Could you check a few things on this model? Use its own coordinates, in mm. A direction names the side the tool comes from. Coordinates: 2 decimals unless noted, no trailing zeros. Write each loop counter-clockwise with the first axis right and the second up, starting at its lowest first coordinate (ties: lowest second). Pieces come first, ordered by that corner, then holes. Notation, with made-up numbers: (82, 39.25) - (93, 39.25) arc R26 ccw to (93, 60.25) - close; hole circle Ø7 at (68.5, -25). An arc over 180 degrees is marked (long way). Write item = value, one per line. Start each with the question number.
```python
from build123d import *

# Parameters (mm, degrees)
BOSS_EXTRUDE1_DEPTH = 2.9972
SKETCH2_R           = 3
BOSS_EXTRUDE2_DEPTH = 11.176
SKETCH3_R           = 4.4958
BOSS_EXTRUDE3_DEPTH = 1.016
CUT_EXTRUDE1_DEPTH  = 1.524
SKETCH5_R           = 3.556
CUT_EXTRUDE2_DEPTH  = 1.9812
SKETCH6_R           = 1.1176
CUT_EXTRUDE3_DEPTH  = 32.262860272
SKETCH9_R           = 0.9906
CUT_EXTRUDE4_DEPTH  = 10.16


with BuildPart() as part:
    # Sketch1 → Boss-Extrude1 (new body)
    with BuildSketch(Plane(origin=(0, 0, 0), x_dir=(0, 0, -1), z_dir=(1, 0, 0))):
        with BuildLine():
            Line((24.769539012, 3.626266444), (5.771274976, 5.288399174))
            ThreePointArc((5.771274976, 5.288399174), (0, 0), (5.771274976, -5.288399174))
            Line((5.771274976, -5.288399174), (24.769539012, -3.626266444))
            ThreePointArc((24.769539012, -3.626266444), (28.0924, 0), (24.769539012, 3.626266444))
        make_face()
    extrude(amount=BOSS_EXTRUDE1_DEPTH)

    # Sketch2 → Boss-Extrude2 (add)
    with BuildSketch(Plane.ZY):
        with Locations(Location((-5.3086, 0, 0), (0, 0, 180))):
            Circle(SKETCH2_R)
    extrude(amount=BOSS_EXTRUDE2_DEPTH)

    # Sketch3 → Boss-Extrude3 (add)
    with BuildSketch(Plane.ZY):
        with Locations(Location((-5.3086, 0, 0), (0, 0, 180))):
            Circle(SKETCH3_R)
    extrude(amount=BOSS_EXTRUDE3_DEPTH)

    # Sketch4 → Cut-Extrude1 (cut)
    with BuildSketch(Plane(origin=(2.9972, 0, 0), x_dir=(0, 0, -1), z_dir=(1, 0, 0))):
        with BuildLine():
            Line((24.703126336, 2.867166085), (5.7048623, 4.529298814))
            ThreePointArc((5.7048623, 4.529298814), (0.762, 0), (5.7048623, -4.529298814))
            Line((5.7048623, -4.529298814), (24.703126336, -2.867166085))
            ThreePointArc((24.703126336, -2.867166085), (27.3304, 0), (24.703126336, 2.867166085))
        make_face()
    extrude(amount=-CUT_EXTRUDE1_DEPTH, mode=Mode.SUBTRACT)

    # Sketch5 → Cut-Extrude2 (cut)
    with BuildSketch(Plane(origin=(1.4732, 0, 0), x_dir=(0, 0, -1), z_dir=(1, 0, 0))):
        with Locations((5.3086, 0)):
            Circle(SKETCH5_R)
    extrude(amount=-CUT_EXTRUDE2_DEPTH, mode=Mode.SUBTRACT)

    # Sketch6 → Cut-Extrude3 (cut, through all)
    with BuildSketch(Plane(origin=(1.4732, 0, 0), x_dir=(0, 0, -1), z_dir=(1, 0, 0))):
        with Locations((21.2344, 0)):
            Circle(SKETCH6_R)
    extrude(amount=-CUT_EXTRUDE3_DEPTH, mode=Mode.SUBTRACT)

    # Sketch9 → Cut-Extrude4 (cut)
    with BuildSketch(Plane(origin=(0, -4.097011229, -7.096231608), x_dir=(-1, 0, 0), z_dir=(0, -0.500000000000004, -0.8660254037844363))):
        with Locations(Location((9.022814295, 2.6543, 0), (0, 0, 90))):
            Circle(SKETCH9_R)
    extrude(amount=-CUT_EXTRUDE4_DEPTH, mode=Mode.SUBTRACT)


solid = part.part
```
1) For P1, Ø4, axis at x = 1.5, z = -23, coming from the -Y side; P2, Ø3, axis at x = -3, z = -18.5, coming from the +Y side; P3, Ø5.5, axis at y = -2, z = -13, coming from the -X side; P4, Ø6, axis at x = 1.5, y = -2, coming from the +Z side, each with a flat end and sliding along its axis, tell me the tip position at first contact or that it passes through.
2) Suppose I cut it at C-C on x = -7.5. Please give me the cut outline in (y, z), plus the area to 3 significant figures.
3) Suppose I cut it at D-D on z = -10.5. Please give me the cut outline in (x, y), plus the area to 3 significant figures.
4) If I drill on probe 1 along Z at (x, y) = (2.1, 0); probe 2 along X at (y, z) = (1.75, -9); probe 3 along X at (y, z) = (4, -9.75), over which ranges is the centre line in solid material (lowest first)? Write a range as [from, to].
5) Suppose I cut it at B-B on y = 0. State how many separate pieces and enclosed holes the cut face has, plus the area to 3 significant figures.
6) Thinking about a two-plate mould opening in X: for faces 1 (the cylindrical face through (-10, 0, -5)), 2 (the cylindrical face through (-0.501, 2.736, -1.741)), 3 (the flat face through (-0.508, 0, -5)), which applies, +X half, -X half, draft (parallel to the pull), parting line (faces both ways), or undercut?
7) Suppose I cut it at A-A on z = -22. Please give me the cut outline in (x, y).
8) Which directions (+Z, -Z, +X, -X, +Y, -Y) give clear straight access to the entire face, cutting with the end or side of a thin tool? Please do faces 4 (the cylindrical face through (-6.02, -2.03, -3.1)), 5 (the flat face through (1.478, 4.446, -15.403)), 6 (the cylindrical face through (2.246, 0.106, -0.763)).
Reply:
q1.P1 = -3.96
q1.P2 = through
q1.P3 = 0
q1.P4 = 0
q2.outline = circle Ø6 at (0, -5.31)
q2.area = 28.3 mm^2
q3.outline = (0, -4.87) - (3, -4.87) - (3, -4.11) - (1.47, -4.11) - (1.47, 4.11) - (3, 4.11) - (3, 4.87) - (0, 4.87) - close
q3.area = 16.7 mm^2
q4.probe_1 = [-28.09, -27.33], [-0.76, 0]
q4.probe_2 = [-1.02, 1.47]
q4.probe_3 = [0, 1.47]
q5.separate_pieces = 2
q5.enclosed_holes = 1
q5.area = 90.3 mm^2
q6.face_1 = undercut
q6.face_2 = draft
q6.face_3 = +X half
q7.outline = (0, -3.87) - (3, -3.87) - (3, -3.1) - (1.47, -3.1) - (1.47, -0.81) - (0, -0.81) - close; (0, 0.81) - (1.47, 0.81) - (1.47, 3.1) - (3, 3.1) - (3, 3.87) - (0, 3.87) - close
q8.face_4 = -X
q8.face_5 = -Z, +X, -X, +Y
q8.face_6 = +X
